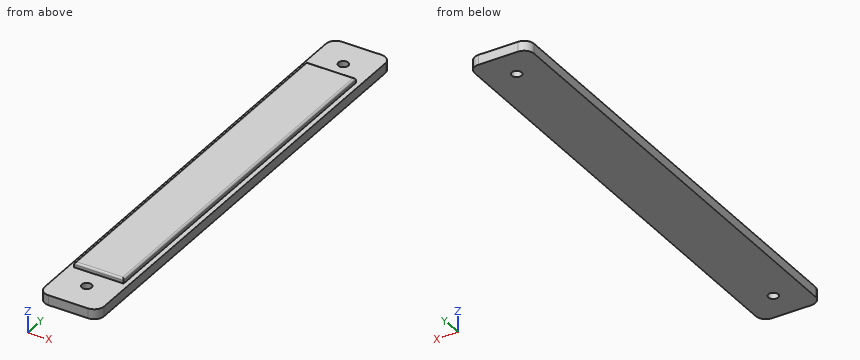
from build123d import *

# Parameters (mm, degrees)
F1_DEPTH = 3.175
F2_D     = 3.175
F3_W     = 15.875
F3_H     = 120.65
F4_DEPTH = 1.5875
F5_R     = 0.635


# Not quite as in the source:
# - a feature names something its author has since deleted; it is built from what else it names


with BuildPart() as f1:
    # F0 (on Top) → F1 (new body)
    with BuildSketch(Plane.XY):
        with BuildLine():
            Line((6.35, 76.2), (-6.35, 76.2))
            ThreePointArc((-6.35, 76.2), (-8.5950640303, 75.2700640303), (-9.525, 73.025))
            Line((-9.525, 73.025), (-9.525, -73.025))
            ThreePointArc((-9.525, -73.025), (-8.5950640303, -75.2700640303), (-6.35, -76.2))
            Line((-6.35, -76.2), (6.35, -76.2))
            ThreePointArc((6.35, -76.2), (8.5950640303, -75.2700640303), (9.525, -73.025))
            Line((9.525, -73.025), (9.525, 73.025))
            ThreePointArc((9.525, 73.025), (8.5950640303, 75.2700640303), (6.35, 76.2))
        make_face()
    extrude(amount=F1_DEPTH)

    # F2 (through all)
    with Locations(Plane(origin=(0, 0, 0), x_dir=(1, 0, 0), z_dir=(0, 0, -1))):
        with Locations((0, 66.675), (0, -66.675)):
            Hole(F2_D / 2)

    # F3 (on face) → F4 (join)
    with BuildSketch(Plane.XY.offset(3.175)):
        Rectangle(F3_W, F3_H)
    extrude(amount=F4_DEPTH)

    # F5
    f5_edges = [f1.edges().sort_by_distance(p)[0] for p in [
        (0, -60.325, 4.7625),
        (7.9375, 0, 4.7625),
        (-7.9375, 0, 4.7625),
        (0, 60.325, 4.7625),
    ]]
    fillet(f5_edges, radius=F5_R)


solid = f1.part
Could you check a few things on this model? Use its own coordinates, in mm. Coordinates: 2 decimals unless noted, no trailing zeros. Loops run counter-clockwise (first coordinate to the right, second up) from the corner with the lowest first, then second, coordinate; pieces in that order, holes last. Notation, with made-up numbers: (60.25, 35.25) -> (90.25, 35.25) arc R12 ccw to (90.25, 41.25) -> close; hole circle Ø11 at (-22, 45.25). An arc over 180 degrees is marked (long way). Answer in a Markdown table with one row per item.
(1) If I drill on probe 1 along Y at (x, z) = (0, 1.85); probe 2 along X at (y, z) = (12, 3.7); probe 3 along Y at (x, z) = (-3.75, 3.8) (3 decimals), over which ranges is the centre line in solid material (lowest first)?
Results found:
| item | result |
|---|---|
| probe 1 | y = -76.2 to -68.26, -65.09 to 65.09, 68.26 to 76.2 |
| probe 2 | x = -7.94 to 7.94 |
| probe 3 | y = -60.325 to 60.325 |
(2) Will these pins go through, and if not, where does the flat tip stop? pin 1 Ø2.5 at (x, y) = (0, 66.675) entering from +Z; pin 2 Ø1 at (y, z) = (28, 4) entering from -X; pin 3 Ø0.5 at (x, z) = (1, 4) entering from +Y (3 decimals); pin 4 Ø1 at (x, z) = (7, 2) entering from -Y.
Results found:
| item | result |
|---|---|
| pin 1 | passes through |
| pin 2 | stops at x = -7.94 |
| pin 3 | stops at y = 60.325 |
| pin 4 | stops at y = -76.2 |
(3) Imagine slicing it at A-A (x = 0). List the corners of the cut face in (y, z) for me (1 decimal), plus the area to 3 significant figures.
Results found:
| item | result |
|---|---|
| outline | (-76.2, 0) -> (-68.3, 0) -> (-68.3, 3.2) -> (-76.2, 3.2) -> close; (-65.1, 0) -> (65.1, 0) -> (65.1, 3.2) -> (60.3, 3.2) -> (60.3, 4.1) arc R0.6 ccw to (59.7, 4.8) -> (-59.7, 4.8) arc R0.6 ccw to (-60.3, 4.1) -> (-60.3, 3.2) -> (-65.1, 3.2) -> close; (68.3, 0) -> (76.2, 0) -> (76.2, 3.2) -> (68.3, 3.2) -> close |
| area | 655 mm^2 |
(4) Imagine slicing it at B-B (y = 50). List the corners of the cut face in (x, z) for me (1 decimal).
Results found:
| item | result |
|---|---|
| outline | (-9.5, 0) -> (9.5, 0) -> (9.5, 3.2) -> (7.9, 3.2) -> (7.9, 4.1) arc R0.6 ccw to (7.3, 4.8) -> (-7.3, 4.8) arc R0.6 ccw to (-7.9, 4.1) -> (-7.9, 3.2) -> (-9.5, 3.2) -> close |
